```python
from build123d import *

# Parameters (mm, degrees)
BASEHEAD_DEPTH  = 4
SKE2_R          = 0.8
HOLE_DEPTH      = 6.773502692
HOLE_DEPTH_BACK = 6.773502692


with BuildPart() as part:
    # BodySke → BaseBody (revolve)
    with BuildSketch(Plane.XY):
        Polygon((0, 0), (0, 3.5), (12.5, 3.5), (13, 3), (22.5, 3), (23.5, 2), (25, 2), (25, 0), align=None)
    revolve(axis=Axis((0, 0, 0), (-1, 0, 0)))

    # Ske → BaseHead (add)
    with BuildSketch(Plane.ZY):
        Polygon((0, 5.773502692), (-5, 2.886751346), (-5, -2.886751346), (0, -5.773502692), (5, -2.886751346), (5, 2.886751346), align=None)
    extrude(amount=BASEHEAD_DEPTH)

    # Ske1 → HeadFillet (revolve, cut)
    with BuildSketch(Plane.XY):
        Polygon((-4, 5.773502692), (-3.72575328, 5.773502692), (-4, 4.75), align=None)
    revolve(axis=Axis((0, 0, 0), (-1, 0, 0)), mode=Mode.SUBTRACT)

    # Ske2 → Hole (cut, two sides)
    with BuildSketch(Plane(origin=(0, 0, 0), x_dir=(1, 0, 0), z_dir=(0, 1, 0))) as hole_sk:
        with Locations((19.5, 0)):
            Circle(SKE2_R)
    extrude(amount=HOLE_DEPTH, mode=Mode.SUBTRACT)
    extrude(hole_sk.sketch, amount=-HOLE_DEPTH_BACK, mode=Mode.SUBTRACT)


solid = part.part
```
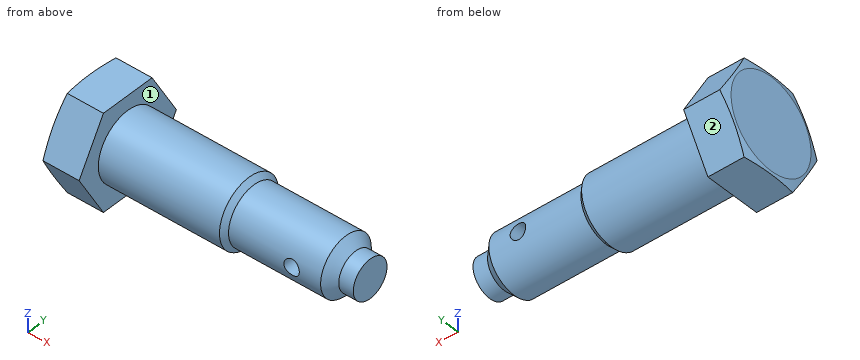
Geometry: final body of the model. Coordinates: model frame, mm. Face numbers are marked on the shaded views. A direction names the side the tool comes from. Coordinates: 2 decimals unless noted, no trailing zeros. Order: outer loops, then holes, each group sorted by start corner. A loop starts at its lowest first (then second) coordinate and runs counter-clockwise, first axis right, second up. Notation, with made-up numbers: M 67.5,-15 L 72.5,-15 A10 ccw 72.5,-3 Z; hole C -29.5,88 d1. An arc over 180 degrees is marked long. Answer in a Markdown table with one row per item. Add a question column.
Q1. Line query: L1, parallel to X at y = -0.75, z = 0; L2, parallel to X at y = -1.5, z = -3.5; L3, parallel to Y at x = 7.25, z = 0. Output: solid intervals per line, ascending.
Q2. Contact query for flat-ended pins moving along their axis: P1, Ø2, axis at x = 18, z = -1.5, coming from the +Y side; P2, Ø6, axis at x = 14.5, y = -4, coming from the +Z side; P3, Ø1, axis at y = -0.5, z = -3.5, coming from the +X side. Output: stop coordinate, or through.
Q3. Reachability of the marked faces 1 and 2 from +Z, -Z, +X, -X, +Y, -Y: full face, straight path, thin tool, end or side. Return the list, or none.
Q4. Section query A-A on x = -0.75. Return the cut outline in (y, z).
Q5. Section query B-B on x = 19.5. Return the cut outline in (y, z).
Q6. Section query C-C on x = 4.75. Return the cut outline in (y, z).
Completed:
| question | item | result |
|---|---|---|
| 1 | L1 | x = -4 to 18.7, 20.3 to 25 |
| 1 | L2 | x = -4 to 0 |
| 1 | L3 | y = -3.5 to 3.5 |
| 2 | P1 | stops at y = 2.96 |
| 2 | P2 | stops at z = 3.02 |
| 2 | P3 | stops at x = 12.96 |
| 3 | face 1 | +X |
| 3 | face 2 | -Z, +X, -X, +Y |
| 4 | outline | M -5.77,0 L -2.89,-5 L 2.89,-5 L 5.77,0 L 2.89,5 L -2.89,5 Z |
| 5 | outline | M -2.89,-0.8 A3 ccw 2.89,-0.8 Z; M -2.89,0.8 L 2.89,0.8 A3 ccw Z |
| 6 | outline | C 0,0 d7 |
